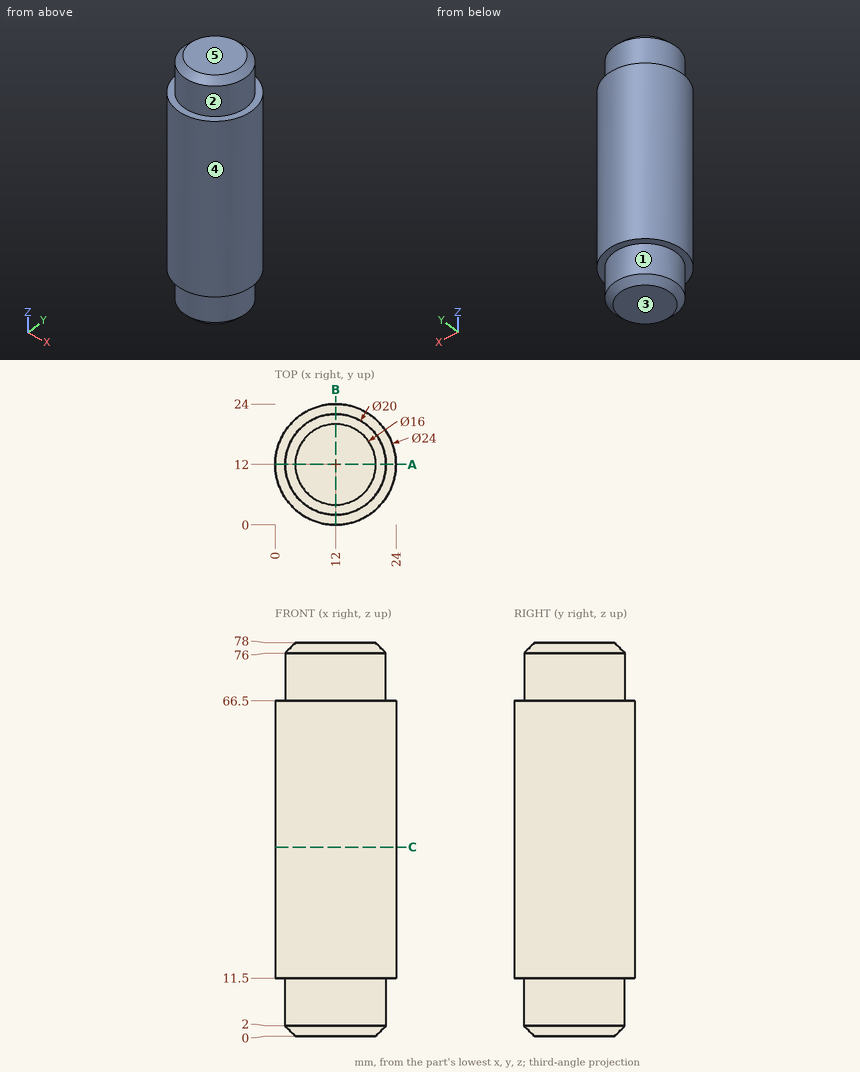
Job drawing, mm, ordinate dimensions from the low corner. One solid piece. A direction names the side the tool comes from. Round coordinates to 2 decimals unless told otherwise and drop trailing zeros. Loops run counter-clockwise (first coordinate to the right, second up) from the corner with the lowest first, then second, coordinate; pieces in that order, holes last.
(1) Wall check: line 1 along Y through (x, z) = (12.25, 44); line 2 along Z through (x, y) = (16.5, 1.75); line 3 along Y through (x, z) = (13.5, 5). Give the ranges that are in metal, low to high.
(2) Cut at C-C (z = 37.5). Give the cut face in (x, y).
(3) Drop flat-ended pins along their axis: pin 1 (8 mm diameter, centred on y = 6, z = 16, fed in from -X); pin 2 (4 mm diameter, centred on y = 10.5, z = 15, fed in from -X); pin 3 (5 mm diameter, centred on y = 9, z = 52.5, fed in from +X); pin 4 (6 mm diameter, centred on x = 17.5, z = 10.5, fed in from -Y). Give the stop position or say it passes through.
(4) Two-plate mould, pull along Z, no slides. Class the marked faces 3, 4 and 5: +Z half, -Z half, draft (parallel to the pull), parting line (faces both ways), or undercut.
(5) Which spindle directions (+Z, -Z, +X, -X, +Y, -Y) get a long thin tool onto all of the face, cutting with end or side? Do the marked faces 1 and 2. Say none if no direction does.
(6) Cut at A-A (y = 12). Give the cut face in (x, z).
Findings below:
1. line 1: y = 0 to 24
1. line 2: z = 11.5 to 66.5
1. line 3: y = 2.11 to 21.89
2. outline: circle Ø24 at (12, 12)
3. pin 1: stops at x = 0.17
3. pin 2: stops at x = 0
3. pin 3: stops at x = 23.99
3. pin 4: stops at y = 0.3
4. face 3: -Z half
4. face 4: draft
4. face 5: +Z half
5. face 1: -Z
5. face 2: +Z
6. outline: (0, 11.5) - (2, 11.5) - (2, 2) - (4, 0) - (20, 0) - (22, 2) - (22, 11.5) - (24, 11.5) - (24, 66.5) - (22, 66.5) - (22, 76) - (20, 78) - (4, 78) - (2, 76) - (2, 66.5) - (0, 66.5) - close
